Geometry check sheet. Reference: the model listing, model coordinates, mm. Face numbers are marked on the shaded views. Give positions to 0.01 mm unless a question says otherwise; leave off trailing zeros. Write each loop counter-clockwise with the first axis right and the second up, starting at its lowest first coordinate (ties: lowest second). Pieces come first, ordered by that corner, then holes. Notation, with made-up numbers: (-35.75, 54.5) -> (10.25, 54.5) arc R18 ccw to (10.25, 86.5) -> close; hole circle Ø8 at (11.5, 14). An arc over 180 degrees is marked (long way). Use a Markdown table: item, result. Add a question column.
from build123d import *

# Parameters (mm, degrees)
F0_R          = 20
F0_R_2        = 15
F1_DEPTH      = 50
F3_R          = 5
F4_DEPTH      = 50
F4_DEPTH_BACK = 4
F6_R          = 10
F7_DEPTH      = 50


with BuildPart() as f1:
    # F0 (on Front) → F1 (new body, symmetric)
    with BuildSketch(Plane.XZ):
        Circle(F0_R)
        Circle(F0_R_2, mode=Mode.SUBTRACT)
    extrude(amount=F1_DEPTH, both=True)

    # F3 (on offset) → F4 (join, two sides)
    with BuildSketch(Plane.XY.offset(-20)) as f4_sk:
        with Locations((0, 30.9999954911)):
            Circle(F3_R)
        with Locations((0, -30.9999954911)):
            Circle(F3_R)
    extrude(amount=-F4_DEPTH)
    extrude(f4_sk.sketch, amount=F4_DEPTH_BACK)

    # F6 (on offset) → F7 (cut)
    with BuildSketch(Plane.YZ.offset(20)):
        Circle(F6_R)
    extrude(amount=-F7_DEPTH, mode=Mode.SUBTRACT)


solid = f1.part
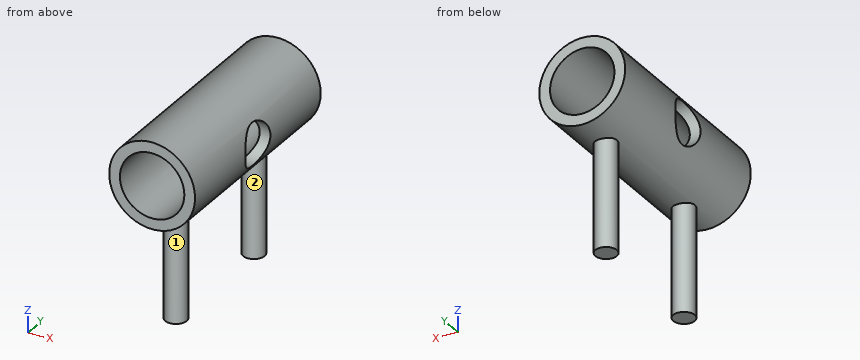
1) Draft check along Y on the marked faces 1 and 2. Enter one of: +Y half, -Y half, draft (parallel to the pull), parting line (faces both ways), or undercut.
2) Sectioned sample at A-A, the plane x = 0. Enter the section's corners in (y, z), and give its area (3 significant figures).
3) Sectioned sample at C-C, the plane z = 0. Enter the section's corners in (x, y).
4) Sectioned sample at B-B, the plane z = 12. Enter the section's corners in (x, y).
5) Sectioned sample at D-D, the plane y = 3.5. Enter the section's corners in (x, z).
6) Material ranges on probe 1 along Z at (x, y) = (0, 12); probe 2 along Y at (x, z) = (-4.5, -64.5); probe 3 along Z at (x, y) = (-6, 21.5), recorded low to high. Write a range as [from, to].
7) Gauge pin test, flat ends, axial feed: P1, Ø4, axis at y = -34.5, z = -38.5, coming from the -X side; P2, Ø2, axis at y = 13, z = 4, coming from the +X side; P3, Ø3, axis at x = -4.5, y = -16, coming from the -Z side. Record the tip position at first contact, or that the pin passes through.
Check values:
| question | item | result |
|---|---|---|
| 1 | face 1 | undercut |
| 1 | face 2 | undercut |
| 2 | outline | (-50, -20) -> (-36, -20) -> (-36, -70) -> (-26, -70) -> (-26, -20) -> (26, -20) -> (26, -70) -> (36, -70) -> (36, -20) -> (50, -20) -> (50, -15) -> (-50, -15) -> close; (-50, 15) -> (50, 15) -> (50, 20) -> (-50, 20) -> close |
| 2 | area | 2,000 mm² |
| 3 | outline | (-20, -50) -> (-15, -50) -> (-15, -10) -> (-20, -10) -> close; (-20, 10) -> (-15, 10) -> (-15, 50) -> (-20, 50) -> close; (15, -50) -> (20, -50) -> (20, -10) -> (15, -10) -> close; (15, 10) -> (20, 10) -> (20, 50) -> (15, 50) -> close |
| 4 | outline | (-16, -50) -> (-9, -50) -> (-9, 50) -> (-16, 50) -> close; (9, -50) -> (16, -50) -> (16, 50) -> (9, 50) -> close |
| 5 | outline | (-17.67, -9.37) arc R20 ccw to (17.67, -9.37) -> (11.72, -9.37) arc R15 cw to (-11.72, -9.37) -> close; (-17.67, 9.37) -> (-11.72, 9.37) arc R15 cw to (11.72, 9.37) -> (17.67, 9.37) arc R20 ccw to start |
| 6 | probe 1 | [-20, -15], [15, 20] |
| 6 | probe 2 | [-33.18, -28.82], [28.82, 33.18] |
| 6 | probe 3 | [-19.08, -13.75], [13.75, 19.08] |
| 7 | P1 | x = -4.77 |
| 7 | P2 | x = 19.77 |
| 7 | P3 | z = -19.77 |
